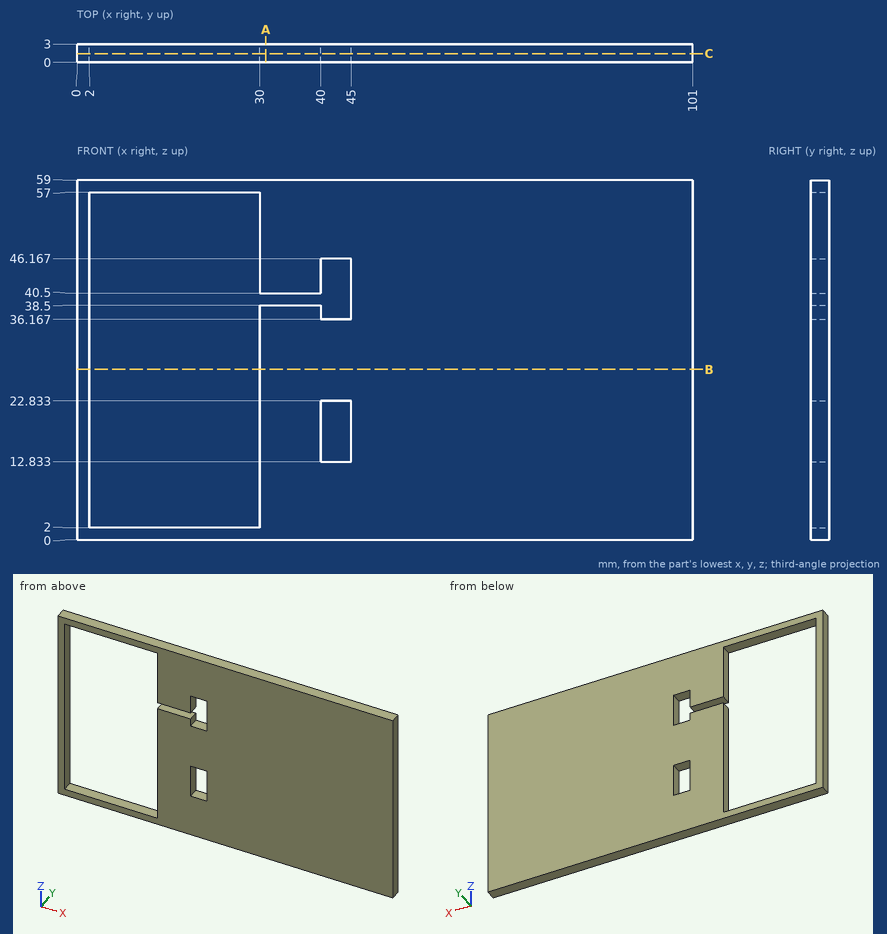
For this review, use the dimensioned drawing (mm, ordinates from the lowest corner) and the shaded views. Coordinates: 2 decimals unless noted, no trailing zeros. Loops run counter-clockwise (first coordinate to the right, second up) from the corner with the lowest first, then second, coordinate; pieces in that order, holes last.
1. Add section B-B, the plane z = 28. Give the boundary of the cut face in (x, y), then the cut area to 3 significant figures.
2. Insertion check: P1, Ø0.9, axis at y = 1.5, z = 43.5, coming from the -X side. The pin has a flat end and moves straight along its axis. Give the tip position at first contact, or say it passes through.
3. Add section C-C, the plane y = 1.4. Give the boundary of the cut face in (x, z).
4. Add section A-A, the plane x = 31. Give the boundary of the cut face in (y, z), then the cut area to 3 significant figures.
5. For line 1 (X direction, y = 0.2, z = 38); line 2 (Z direction, x = 42.5, y = 2.75); line 3 (X direction, y = 2.85, z = 30.5), list the stretches that pass through material, from the lowest coordinate up.
Result:
1. outline: (0, 0) - (2, 0) - (2, 3) - (0, 3) - close; (30, 0) - (101, 0) - (101, 3) - (30, 3) - close
1. area: 219 mm2
2. P1: stops at x = 0
3. outline: (0, 0) - (101, 0) - (101, 59) - (0, 59) - close; hole (2, 2) - (30, 2) - (30, 38.5) - (40, 38.5) - (40, 36.17) - (45, 36.17) - (45, 46.17) - (40, 46.17) - (40, 40.5) - (30, 40.5) - (30, 57) - (2, 57) - close; hole (40, 12.83) - (45, 12.83) - (45, 22.83) - (40, 22.83) - close
4. outline: (0, 0) - (3, 0) - (3, 38.5) - (0, 38.5) - close; (0, 40.5) - (3, 40.5) - (3, 59) - (0, 59) - close
4. area: 171 mm2
5. line 1: x = 0 to 2, 30 to 40, 45 to 101
5. line 2: z = 0 to 12.83, 22.83 to 36.17, 46.17 to 59
5. line 3: x = 0 to 2, 30 to 101
